Input: part model. Units: mm. Frame: model coordinates. Face numbers are marked on the shaded views. A direction names the side the tool comes from. Give positions to 0.01 mm unless a question says otherwise; leave off trailing zeros. Loops run counter-clockwise (first coordinate to the right, second up) from the corner with the lowest first, then second, coordinate; pieces in that order, holes last. Notation, with made-up numbers: (77.25, 69) - (119.25, 69) arc R19 ccw to (119.25, 105) - close; hole circle Ø9 at (7.5, 75). An arc over 180 degrees is marked (long way). Answer as a JSON object with one key per item and string values.
from build123d import *

# Parameters (mm, degrees)
MODEL_R                 = 1.5
SALIENTE_EXTRUIR1_DEPTH = 3


with BuildPart() as part:
    # Model → Saliente-Extruir1 (new body)
    with BuildSketch(Plane.XY):
        with BuildLine():
            Line((110.375172306, 212.589330986), (110.375172306, 211.089330986))
            Line((110.375172306, 211.089330986), (107.375172306, 211.089330986))
            Line((107.375172306, 211.089330986), (107.375172306, 209.23522902))
            ThreePointArc((107.375172306, 209.23522902), (108.769472902, 208.385555371), (110.375172306, 208.089330986))
            Line((110.375172306, 208.089330986), (114.125172656, 208.089330986))
            ThreePointArc((114.125172656, 208.089330986), (114.655502742, 207.869661072), (114.875172656, 207.339330986))
            Line((114.875172656, 207.339330986), (114.875172656, 205.839330986))
            ThreePointArc((114.875172656, 205.839330986), (114.655502742, 205.3090009), (114.125172656, 205.089330986))
            Line((114.125172656, 205.089330986), (110.375172306, 205.089330986))
            ThreePointArc((110.375172306, 205.089330986), (107.192564198, 203.770683786), (105.875172656, 200.587555713))
            Line((105.875172656, 200.587555713), (105.875172656, 181.089330986))
            Line((105.875172656, 181.089330986), (110.375172306, 181.089330986))
            Line((110.375172306, 181.089330986), (110.375172306, 179.589330986))
            Line((110.375172306, 179.589330986), (137.375172656, 179.589330986))
            Line((137.375172656, 179.589330986), (137.375172656, 181.089330986))
            Line((137.375172656, 181.089330986), (141.875172656, 181.089330986))
            Line((141.875172656, 181.089330986), (141.875172306, 200.589330986))
            ThreePointArc((141.875172306, 200.589330986), (140.554536331, 203.773925842), (137.367774797, 205.089324906))
            Line((137.367774797, 205.089324906), (133.625176703, 205.089319857))
            ThreePointArc((133.625176703, 205.089319857), (133.09484632, 205.308989056), (132.875175691, 205.839318846))
            Line((132.875175691, 205.839318846), (132.875173667, 207.339318846))
            ThreePointArc((132.875173667, 207.339318846), (133.094842866, 207.869649228), (133.625172656, 208.089319857))
            Line((133.625172656, 208.089319857), (137.375178726, 208.089324916))
            ThreePointArc((137.375178726, 208.089324916), (138.980875531, 208.385553219), (140.375172656, 209.23522902))
            Line((140.375172656, 209.23522902), (140.375172656, 211.089330986))
            Line((140.375172656, 211.089330986), (137.375172656, 211.089330986))
            Line((137.375172656, 211.089330986), (137.375165869, 212.589324916))
            Line((137.375165869, 212.589324916), (110.375172306, 212.589330986))
        make_face()
        with Locations((110.375172306, 185.589330986)):
            Circle(MODEL_R, mode=Mode.SUBTRACT)
        with Locations((119.375172306, 185.589330986)):
            Circle(MODEL_R, mode=Mode.SUBTRACT)
        with Locations((110.375172306, 194.589330986)):
            Circle(MODEL_R, mode=Mode.SUBTRACT)
        with Locations((119.375172306, 194.589330986)):
            Circle(MODEL_R, mode=Mode.SUBTRACT)
        with Locations((128.375172306, 185.589330986)):
            Circle(MODEL_R, mode=Mode.SUBTRACT)
        with Locations((137.375172306, 185.589330986)):
            Circle(MODEL_R, mode=Mode.SUBTRACT)
        with Locations((128.375172306, 194.589330986)):
            Circle(MODEL_R, mode=Mode.SUBTRACT)
        with Locations((137.375172306, 194.589330986)):
            Circle(MODEL_R, mode=Mode.SUBTRACT)
        with Locations((119.375172656, 203.589330986)):
            Circle(MODEL_R, mode=Mode.SUBTRACT)
        with Locations((128.375172656, 203.589330986)):
            Circle(MODEL_R, mode=Mode.SUBTRACT)
    extrude(amount=SALIENTE_EXTRUIR1_DEPTH)


solid = part.part
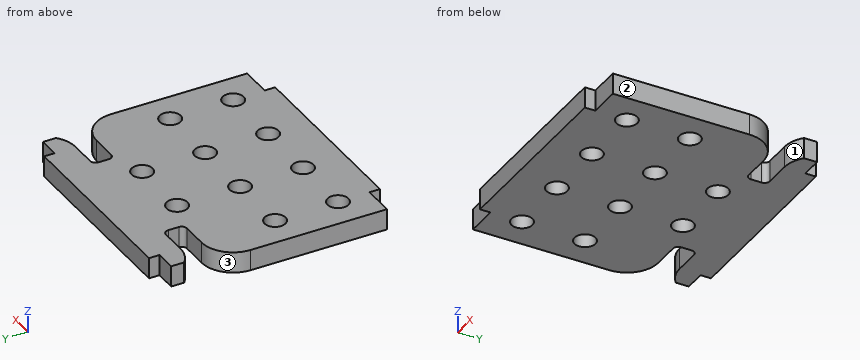
Item 1: Material intervals for line 1 (X direction, y = 194.5, z = 2.05); line 2 (X direction, y = 194, z = 1.85); line 3 (Y direction, x = 129, z = 2.7), sorted ascending. Write a range as [from, to].
Geometry check:
{"line 1": "x = [105.88, 108.88], [111.87, 117.88], [120.87, 126.88], [129.87, 135.88], [138.87, 141.88]", "line 2": "x = [105.88, 109], [111.75, 118], [120.75, 127], [129.75, 136], [138.75, 141.88]", "line 3": "y = [179.59, 184.23], [186.95, 193.23], [195.95, 202.23], [204.95, 212.59]"}
Item 2: Cut plane D-D (z = 1.75). Give the number of separate pieces and of enclosed holes in the cut face, then the cut area to 3 significant figures.
Geometry check:
{"separate pieces": "1", "enclosed holes": "10", "area": "1,020 mm2"}
Item 3: Cut plane B-B (y = 186). Return loops of the section in (x, z), then the cut area to 3 significant figures.
Geometry check:
{"outline": "(105.88, 0) - (108.93, 0) - (108.93, 3) - (105.88, 3) - close; (111.82, 0) - (117.93, 0) - (117.93, 3) - (111.82, 3) - close; (120.82, 0) - (126.93, 0) - (126.93, 3) - (120.82, 3) - close; (129.82, 0) - (135.93, 0) - (135.93, 3) - (129.82, 3) - close; (138.82, 0) - (141.88, 0) - (141.88, 3) - (138.82, 3) - close", "area": "73.4 mm2"}
Item 4: Cut plane A-A (x = 118.5). Return loops of the section in (y, z), then the cut area to 3 significant figures.
Geometry check:
{"outline": "(179.59, 0) - (184.37, 0) - (184.37, 3) - (179.59, 3) - close; (186.81, 0) - (193.37, 0) - (193.37, 3) - (186.81, 3) - close; (195.81, 0) - (202.37, 0) - (202.37, 3) - (195.81, 3) - close; (204.81, 0) - (212.59, 0) - (212.59, 3) - (204.81, 3) - close", "area": "77.1 mm2"}
Item 5: Access query for the marked faces 1, 2 and 3. Directions: +Z, -Z, +X, -X, +Y, -Y. A direction counts if a zero-diameter tool reaches every point of the face in a straight line with its end or side. Return the directions, or none.
Geometry check:
{"face 1": "+Z, -Z, +X", "face 2": "+Z, -Z, +X, +Y, -Y", "face 3": "+Z, -Z, -X"}
Item 6: Contact query for flat-ended pins moving along their axis: P1, Ø0.9, axis at x = 139.5, z = 2, coming from the -Y side; P2, Ø0.6, axis at y = 210.5, z = 2, coming from the -X side; P3, Ø1.2, axis at y = 206.5, z = 1.5, coming from the -X side. Output: stop coordinate, or through.
Geometry check:
{"P1": "stops at y = 181.09", "P2": "stops at x = 107.38", "P3": "stops at x = 114.88"}
Item 7: Cut plane C-C (y = 210). Return loops of the section in (x, z), then the cut area to 3 significant figures.
Geometry check:
{"outline": "(107.38, 0) - (140.38, 0) - (140.38, 3) - (107.38, 3) - close", "area": "99.0 mm2"}
